```python
from build123d import *

# Parameters (mm, degrees)
SKETCH_1_R      = 3.4
SKETCH_1_W      = 6.15
SKETCH_1_H      = 6.15
EXTRUDE_1_DEPTH = 100


with BuildPart() as part:
    # 草图1 → 凸台-拉伸1 (new body)
    with BuildSketch(Plane.XY):
        with BuildLine():
            Line((-4.068782805, 19.545792426), (-17.968782805, 19.545792426))
            ThreePointArc((-17.968782805, 19.545792426), (-18.675889586, 19.252899208), (-18.968782805, 18.545792426))
            Line((-18.968782805, 18.545792426), (-18.968782805, 4.645792426))
            Line((-18.968782805, 4.645792426), (-18.968782805, -5.554207574))
            Line((-18.968782805, -5.554207574), (-18.968782805, -19.454207574))
            ThreePointArc((-18.968782805, -19.454207574), (-18.675889586, -20.161314355), (-17.968782805, -20.454207574))
            Line((-17.968782805, -20.454207574), (20.031217195, -20.454207574))
            ThreePointArc((20.031217195, -20.454207574), (20.738323976, -20.161314355), (21.031217195, -19.454207574))
            Line((21.031217195, -19.454207574), (21.031217195, -5.554207574))
            Line((21.031217195, -5.554207574), (20.031217195, -5.554207574))
            Line((20.031217195, -5.554207574), (20.031217195, -4.554207574))
            Line((20.031217195, -4.554207574), (17.231217195, -4.554207574))
            Line((17.231217195, -4.554207574), (17.231217195, -5.554207574))
            Line((17.231217195, -5.554207574), (19.231217195, -5.554207574))
            Line((19.231217195, -5.554207574), (19.231217195, -10.704207574))
            Line((19.231217195, -10.704207574), (12.483298723, -10.704207574))
            Line((12.483298723, -10.704207574), (8.731217195, -6.952126046))
            Line((8.731217195, -6.952126046), (8.731217195, 6.043710898))
            Line((8.731217195, 6.043710898), (12.483298723, 9.795792426))
            Line((12.483298723, 9.795792426), (19.231217195, 9.795792426))
            Line((19.231217195, 9.795792426), (19.231217195, 4.645792426))
            Line((19.231217195, 4.645792426), (17.231217195, 4.645792426))
            Line((17.231217195, 4.645792426), (17.231217195, 3.645792426))
            Line((17.231217195, 3.645792426), (20.031217195, 3.645792426))
            Line((20.031217195, 3.645792426), (20.031217195, 4.645792426))
            Line((20.031217195, 4.645792426), (21.031217195, 4.645792426))
            Line((21.031217195, 4.645792426), (21.031217195, 18.545792426))
            ThreePointArc((21.031217195, 18.545792426), (20.738323976, 19.252899208), (20.031217195, 19.545792426))
            Line((20.031217195, 19.545792426), (6.131217195, 19.545792426))
            Line((6.131217195, 19.545792426), (6.131217195, 18.545792426))
            Line((6.131217195, 18.545792426), (5.131217195, 18.545792426))
            Line((5.131217195, 18.545792426), (5.131217195, 15.745792426))
            Line((5.131217195, 15.745792426), (6.131217195, 15.745792426))
            Line((6.131217195, 15.745792426), (6.131217195, 17.745792426))
            Line((6.131217195, 17.745792426), (11.281217195, 17.745792426))
            Line((11.281217195, 17.745792426), (11.281217195, 10.997873954))
            Line((11.281217195, 10.997873954), (7.529135667, 7.245792426))
            Line((7.529135667, 7.245792426), (-5.466701277, 7.245792426))
            Line((-5.466701277, 7.245792426), (-9.218782805, 10.997873954))
            Line((-9.218782805, 10.997873954), (-9.218782805, 17.745792426))
            Line((-9.218782805, 17.745792426), (-4.068782805, 17.745792426))
            Line((-4.068782805, 17.745792426), (-4.068782805, 15.745792426))
            Line((-4.068782805, 15.745792426), (-3.068782805, 15.745792426))
            Line((-3.068782805, 15.745792426), (-3.068782805, 18.545792426))
            Line((-3.068782805, 18.545792426), (-4.068782805, 18.545792426))
            Line((-4.068782805, 18.545792426), (-4.068782805, 19.545792426))
        make_face()
        with Locations((1.031217195, -0.454207574)):
            Circle(SKETCH_1_R, mode=Mode.SUBTRACT)
        with Locations((-14.093782805, 14.670792426)):
            Rectangle(SKETCH_1_W, SKETCH_1_H, mode=Mode.SUBTRACT)
        Polygon((-6.668782805, 6.043710898), (-6.668782805, -6.952126046), (-10.420864333, -10.704207574), (-17.168782805, -10.704207574), (-17.168782805, 9.795792426), (-10.420864333, 9.795792426), align=None, mode=Mode.SUBTRACT)
        Polygon((-5.466701277, -8.154207574), (7.529135667, -8.154207574), (11.281217195, -11.906289102), (11.281217195, -18.654207574), (-9.218782805, -18.654207574), (-9.218782805, -11.906289102), align=None, mode=Mode.SUBTRACT)
        with Locations((16.156217195, 14.670792426)):
            Rectangle(SKETCH_1_W, SKETCH_1_H, mode=Mode.SUBTRACT)
        with Locations((-14.093782805, -15.579207574)):
            Rectangle(SKETCH_1_W, SKETCH_1_H, mode=Mode.SUBTRACT)
        with Locations((16.156217195, -15.579207574)):
            Rectangle(SKETCH_1_W, SKETCH_1_H, mode=Mode.SUBTRACT)
    extrude(amount=EXTRUDE_1_DEPTH)


solid = part.part
```
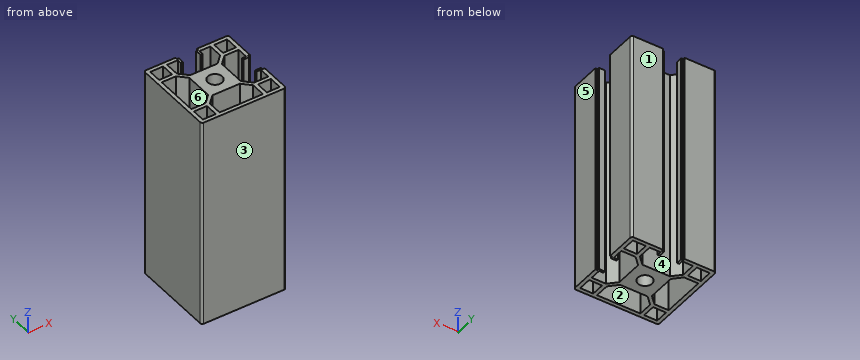
Check sheet for the modelled part. Datum: model origin and axes. Units: mm. Face numbers are marked on the shaded views. A direction names the side the tool comes from. Coordinates: 2 decimals unless noted, no trailing zeros. Write each loop counter-clockwise with the first axis right and the second up, starting at its lowest first coordinate (ties: lowest second). Pieces come first, ordered by that corner, then holes. Notation, with made-up numbers: M 86.5,-35.5 L 102.5,-35.5 A22 ccw 102.5,-9.5 Z; hole C -37,58 d3. An arc over 180 degrees is marked long. Write item = value, one per line. Start each with the question number.
1. Tool access check on the marked faces 1 and 2. Record the directions out of +Z, -Z, +X, -X, +Y, -Y that give a thin tool (end or side, any length) a straight path to the whole face; none if there is none.
2. Sectioned sample at C-C (x = -0.5). Record the cut outline in (y, z).
3. Mould release check, pull along X, two halves, no side actions. Record for the marked faces 3, 4, 5 and 6: pulls with the +X half, pulls with the -X half, needs draft (parallel to the pull), parting line crosses it, or undercut.
4. Go/stop test with flat-tipped pins: pin 1 (0.5 mm diameter, centred on x = 5.5, z = 68, fed in from +Y); pin 2 (1.1 mm diameter, centred on x = 20.5, z = 49.5, fed in from +Y); pin 3 (0.8 mm diameter, centred on y = -5, z = 50, fed in from +X). Record where each tip stops, or that it passes through.
5. Sectioned sample at B-B (x = -14.5). Record the cut outline in (y, z).
6. Sectioned sample at A-A (y = -17.5). Record the cut outline in (x, z), then the cut area to 3 significant figures.
7. Thickness scan on probe 1 along X at (y, z) = (15.5, 14.5); probe 2 along X at (y, z) = (17, 6); probe 3 along Y at (x, z) = (17, 92.5). Record the ranges inside material, lowest first.
8. Sectioned sample at D-D (z = 77.5). State how many separate pieces and enclosed holes the cut face has, then the cut area to 3 significant figures.
The answers:
q1.face_1 = +Z, -Z, +X, -X, +Y
q1.face_2 = +Z, -Z
q2.outline = M -20.45,0 L -18.65,0 L -18.65,100 L -20.45,100 Z; M -8.15,0 L -3.49,0 L -3.49,100 L -8.15,100 Z; M 2.58,0 L 7.25,0 L 7.25,100 L 2.58,100 Z
q3.face_3 = needs draft
q3.face_4 = undercut
q3.face_5 = pulls with the +X half
q3.face_6 = undercut
q4.pin_1 = 18.55
q4.pin_2 = 19.55
q4.pin_3 = 20.03
q5.outline = M -20.45,0 L -18.65,0 L -18.65,100 L -20.45,100 Z; M -12.5,0 L -10.7,0 L -10.7,100 L -12.5,100 Z; M 9.8,0 L 11.6,0 L 11.6,100 L 9.8,100 Z; M 17.75,0 L 19.55,0 L 19.55,100 L 17.75,100 Z
q6.outline = M -18.97,0 L -17.17,0 L -17.17,100 L -18.97,100 Z; M -11.02,0 L -9.22,0 L -9.22,100 L -11.02,100 Z; M 11.28,0 L 13.08,0 L 13.08,100 L 11.28,100 Z; M 19.23,0 L 21.03,0 L 21.03,100 L 19.23,100 Z
q6.area = 720 mm²
q7.probe_1 = -18.97 to -17.17, -11.02 to -9.22, 11.28 to 13.08, 19.23 to 21.03
q7.probe_2 = -18.97 to -17.17, -11.02 to -9.22, -4.07 to -3.07, 5.13 to 6.13, 11.28 to 13.08, 19.23 to 21.03
q7.probe_3 = -20.45 to -18.65, -12.5 to -10.7, 9.8 to 11.6, 17.75 to 19.55
q8.separate_pieces = 1
q8.enclosed_holes = 7
q8.area = 581 mm²
